Source: CAD feature listing. Evaluate the final solid. Frame: model axes, mm. Face numbers are marked on the shaded views. Round coordinates to 2 decimals unless told otherwise and drop trailing zeros. Order: outer loops, then holes, each group sorted by start corner. A loop starts at its lowest first (then second) coordinate and runs counter-clockwise, first axis right, second up. Notation, with made-up numbers: (49.25, -0.75) -> (81.25, -0.75) arc R24 cw to (81.25, 29.25) -> close; hole circle Ø10 at (18, 80.5). An arc over 180 degrees is marked (long way). Use a Markdown table: item, result. Add a question column.
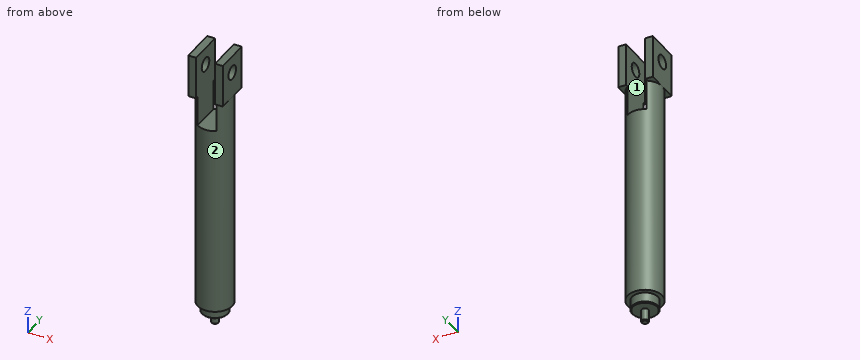
Solid Edge part; units mm, degrees
sketch "Sketch1" plane through (0, 0, 0) normal (0, 0, 1) x (1, 0, 0)
  circle A0 centre (0, 0) radius 20
extrude "Protrusion1" add sketch "Sketch1" along normal blind 340
sketch "Sketch2" plane through (0, 0, 0) normal (0, 0, -1) x (-1, 0, 0)
  circle A0 centre (0, 0) radius 15
  circle A1 centre (0, 0) radius 20
extrude "ExtrudedCutout_12" cut sketch "Sketch2" against normal blind 32.7
sketch "Sketch3" plane through (0, 0, 0) normal (0, 0, -1) x (0, -1, 0)
  circle A0 centre (0, 0) radius 4
  circle A1 centre (0, 0) radius 15
extrude "ExtrudedCutout_13" cut sketch "Sketch3" against normal blind 20.7
sketch "Sketch4" plane through (0, 0, 0) normal (0, 0, -1) x (0, -1, 0)
  circle A0 centre (0, 0) radius 4
extrude "ExtrudedCutout_14" cut sketch "Sketch4" against normal blind 6.2
cosmetic_thread "Thread1"
sketch "Sketch5" plane through (0, 0, 0) normal (0, 1, 0) x (-1, 0, 0)
  line L0 (3, 6.2) -> (4, 7.2)
  line L1 (4, 7.2) -> (4, 6.2)
  line L2 (4, 6.2) -> (3, 6.2)
  line L3 (14, 20.7) -> (15, 20.7)
  line L4 (15, 20.7) -> (15, 21.7)
  line L5 (15, 21.7) -> (14, 20.7)
revolve "RevolvedCutout1" cut sketch "Sketch5" angle 360 about axis through (0, 0, 0) along (0, 0, 1)
sketch "Sketch6" plane through (20, 0, 315) normal (1, 0, 0) x (0, 1, 0)
  circle A0 centre (0, 5) radius 11
extrude "Cutout1" cut sketch "Sketch6" against normal blind 1
sketch "Sketch7" plane through (-20, 0, 315) normal (-1, 0, 0) x (0, -1, 0)
  circle A0 centre (0, 5) radius 11
extrude "ExtrudedCutout_19" cut sketch "Sketch7" against normal blind 1
sketch "Sketch8" plane through (15.5, 0, 340) normal (0, 0, 1) x (0, -1, 0)
  line L0 (-20, -35.5) -> (20, -35.5)
  line L1 (20, -35.5) -> (20, 4.5)
  line L2 (20, 4.5) -> (-20, 4.5)
  line L3 (-20, 4.5) -> (-20, -35.5)
extrude "ExtrudedCutout_21" add sketch "Sketch8" against normal blind 50
sketch "Sketch9" plane through (10, 0.0037, 292.5417) normal (-1, 0, 0) x (0, -1, 0)
  circle A0 centre (0.0037, 27.4583) radius 8
extrude "ExtrudedCutout_5" cut sketch "Sketch9" along normal mid plane 178.997
sketch "Sketch10" plane through (0, -20, 315) normal (0, -1, 0) x (0, 0, -1)
  line L0 (60, 11) -> (-25, 11)
  line L1 (-25, -11) -> (-25, 11)
  line L2 (60, -11) -> (-25, -11)
  line L3 (60, 11) -> (60, -11)
extrude "ExtrudedCutout_20" cut sketch "Sketch10" against normal blind 40
properties material "Steel - Stainless:1.4301 , X5CrNi18-10"
1) Section C-C on z = 210. Output: boundary loops of the cut face in (x, y), then the cut area to 3 significant figures.
2) Section A-A on z = 298. Output: boundary loops of the cut face in (x, y), then the cut area to 3 significant figures.
3) First-contact query: pin 1 Ø2.5 at (x, y) = (16, -7.5) entering from -Z; pin 2 Ø10 at (x, y) = (14.5, 11.5) entering from -Z; pin 3 Ø3 at (y, z) = (12.5, 187.5) entering from -X; pin 4 Ø13 at (y, z) = (0, 320) entering from -X. Flat tips, straight axial feed; report the tip coordinate or a pass-through.
4) Draft query along X for the marked faces 1 and 2. Return one class per face: pulls with the +X half, pulls with the -X half, needs draft (parallel to the pull), parting line crosses it, or undercut.
5) Section B-B on x = 0. Output: boundary loops of the cut face in (y, z).
6) Line query: probe 1 along Z at (x, y) = (13, 0); probe 2 along X at (y, z) = (14, 292); probe 3 along Y at (x, z) = (-17.5, 320). Output: solid intervals per line, ascending. Write a range as from..to.
Conclusion:
| question | item | result |
|---|---|---|
| 1 | outline | circle Ø40 at (0, 0) |
| 1 | area | 1,260 mm^2 |
| 2 | outline | (-20, -20) -> (-11, -20) -> (-11, 20) -> (-20, 20) -> close; (11, -20) -> (20, -20) -> (20, 20) -> (11, 20) -> close |
| 2 | area | 720 mm^2 |
| 3 | pin 1 | stops at z = 32.7 |
| 3 | pin 2 | stops at z = 20.7 |
| 3 | pin 3 | stops at x = -16.7 |
| 3 | pin 4 | passes through |
| 4 | face 1 | undercut |
| 4 | face 2 | parting line crosses it |
| 5 | outline | (-20, 32.7) -> (-15, 32.7) -> (-15, 21.7) -> (-14, 20.7) -> (-4, 20.7) -> (-4, 7.2) -> (-3, 6.2) -> (3, 6.2) -> (4, 7.2) -> (4, 20.7) -> (14, 20.7) -> (15, 21.7) -> (15, 32.7) -> (20, 32.7) -> (20, 255) -> (-20, 255) -> close |
| 6 | probe 1 | z = 20.7..312, 328..340 |
| 6 | probe 2 | x = -20..-11, 11..20 |
| 6 | probe 3 | y = -20..-8, 8..20 |
